The listing builds one solid part. Answer for the finished solid, in the listing's coordinates (mm). A direction names the side the tool comes from. Give positions to 0.01 mm unless a question says otherwise; leave off trailing zeros. Order: outer loops, then holes, each group sorted by start corner. A loop starts at its lowest first (then second) coordinate and runs counter-clockwise, first axis right, second up. Notation, with made-up numbers: (13.5, 73.5) - (59.5, 73.5) arc R17 ccw to (59.5, 78.5) - close; hole circle Ø8 at (39, -26.75). An arc over 180 degrees is marked (long way). Answer in a Markdown table with one row per item.
from build123d import *

# Parameters (mm, degrees)
F0_W     = 4.5
F0_H     = 6
F1_DEPTH = 5
F2_R     = 1.5
F3_DEPTH = 25
F4_W     = 2.115136
F4_H     = 22.957688
F5_DEPTH = 5
F6_R     = 1.5
F7_DEPTH = 25


with BuildPart() as f1:
    # F0 (on Front) → F1 (new body)
    with BuildSketch(Plane.XZ):
        with BuildLine():
            ThreePointArc((0, -11.5), (-8.884864, 0), (0, 11.5))
            Line((0, 11.5), (0, 17.478844))
            Line((0, 17.478844), (-2, 17.478844))
            Line((-2, 17.478844), (-2, 11.478844))
            Line((-2, 11.478844), (-6.5, 11.478844))
            Line((-6.5, 11.478844), (-11, 11.478844))
            Line((-11, 11.478844), (-11, -11.513906))
            Line((-11, -11.513906), (-6.5, -11.513906))
            Line((-6.5, -11.513906), (-2, -11.513906))
            Line((-2, -11.513906), (-2, -17.513906))
            Line((-2, -17.513906), (0, -17.513906))
            Line((0, -17.513906), (0, -11.5))
        make_face()
        with Locations((-4.25, 14.478844)):
            Rectangle(F0_W, F0_H)
        with Locations((-4.25, -14.513906)):
            Rectangle(F0_W, F0_H)
    extrude(amount=F1_DEPTH)

    # F2 (on face) → F3 (cut)
    with BuildSketch(Plane.YZ):
        with Locations((-2.5, 14.478844)):
            Circle(F2_R)
        with Locations((-2.5, -14.513906)):
            Circle(F2_R)
    extrude(amount=-F3_DEPTH, mode=Mode.SUBTRACT)

    # F4 (on face) → F5 (join)
    with BuildSketch(Plane.XZ.offset(5)):
        with Locations((-9.942432, 0)):
            Rectangle(F4_W, F4_H)
    extrude(amount=F5_DEPTH)

    # F6 (on face) → F7 (cut)
    with BuildSketch(Plane(origin=(-11, 0, 0), x_dir=(0, -1, 0), z_dir=(-1, 0, 0))):
        with Locations((7.5, 7.498844)):
            Circle(F6_R)
        with Locations((7.5, -7.501156)):
            Circle(F6_R)
    extrude(amount=-F7_DEPTH, mode=Mode.SUBTRACT)


solid = f1.part
Item 1: Consider line 1 (Z direction, x = -4.5, y = -2); line 2 (Y direction, x = -8, z = 5); line 3 (Z direction, x = -10, y = -3.25). Determine where each line is inside the solid, lowest interval first.
Answer block:
| item | result |
|---|---|
| line 1 | -17.51 to -15.93, -13.1 to -9.22, 9.22 to 13.06, 15.89 to 17.48 |
| line 2 | -5 to 0 |
| line 3 | -11.51 to 11.48 |
Item 2: Find section B-B on z = -8.5. Write down the section's boundary in (x, y).
Answer block:
| item | result |
|---|---|
| outline | (-11, -10) - (-8.88, -10) - (-8.88, -8.62) - (-11, -8.62) - close; (-11, -6.38) - (-8.88, -6.38) - (-8.88, -5) - (-5.31, -5) - (-5.31, 0) - (-11, 0) - close |
Item 3: Find section A-A on y = -7.5. Write down the section's boundary in (x, z).
Answer block:
| item | result |
|---|---|
| outline | (-11, -11.48) - (-8.88, -11.48) - (-8.88, -9) - (-11, -9) - close; (-11, -6) - (-8.88, -6) - (-8.88, 6) - (-11, 6) - close; (-11, 9) - (-8.88, 9) - (-8.88, 11.48) - (-11, 11.48) - close |
Item 4: Each of these flat-tipped pins is pushed along its axis until it touches: P1, Ø2.5, axis at x = -10.5, y = -7.5, coming from the -Z side; P2, Ø4, axis at y = -7.5, z = 2, coming from the +X side; P3, Ø1.3, axis at x = -8.5, y = -3, coming from the +Z side. Where does it stop, or does it pass through?
Answer block:
| item | result |
|---|---|
| P1 | z = -11.48 |
| P2 | x = -8.88 |
| P3 | z = 11.48 |
Item 5: Which of the six approach directions +Z, -Z, +X, -X, +Y, -Y give full straight-line access (tool end or side, diameter ignored) to faces 5 (the face through (-8.885, -7, 0)), 6 (the face through (-10, -10, 0)), 7 (the face through (-10, -7, -11.479))?
Answer block:
| item | result |
|---|---|
| face 5 | +Z, -Z, +X, -Y |
| face 6 | +Z, -Z, +X, -X, -Y |
| face 7 | -Z, +X, -X, -Y |
Item 6: Find section C-C on y = -2.5. Write down the section's boundary in (x, z).
Answer block:
| item | result |
|---|---|
| outline | (-11, -11.51) - (-6.5, -11.51) - (-6.5, -13.01) - (0, -13.01) - (0, -11.5) arc R11.88 cw to (0, 11.5) - (0, 12.98) - (-6.5, 12.98) - (-6.5, 11.48) - (-11, 11.48) - close; (-6.5, -17.51) - (0, -17.51) - (0, -16.01) - (-6.5, -16.01) - close; (-6.5, 15.98) - (0, 15.98) - (0, 17.48) - (-6.5, 17.48) - close |
Item 7: Find section D-D on z = 9.5. Write down the section's boundary in (x, y), then the cut area to 3 significant figures.
Answer block:
| item | result |
|---|---|
| outline | (-11, -10) - (-8.88, -10) - (-8.88, -5) - (-4.14, -5) - (-4.14, 0) - (-11, 0) - close |
| area | 44.9 mm² |
Item 8: Determine the mould class of faces 1 (the face through (-9, -4, 11.479)), 2 (the face through (-8.883, -2.465, -0.219)), 3 (the face through (-5, -5, 13)), 4 (the face through (-9, -2, -11.514)) for opening direction Z: pulls with the +Z half, pulls with the -Z half, needs draft (parallel to the pull), parting line crosses it, or undercut.
Answer block:
| item | result |
|---|---|
| face 1 | pulls with the +Z half |
| face 2 | undercut |
| face 3 | needs draft |
| face 4 | pulls with the -Z half |
